Geometry check sheet. Reference: the model listing, model coordinates, mm. A direction names the side the tool comes from. Round coordinates to 2 decimals unless told otherwise and drop trailing zeros. Order: outer loops, then holes, each group sorted by start corner. A loop starts at its lowest first (then second) coordinate and runs counter-clockwise, first axis right, second up. Notation, with made-up numbers: (89.25, -24.75) - (139.25, -24.75) arc R21 cw to (139.25, -12.75) - close; hole circle Ø11 at (34.5, 39.25). An arc over 180 degrees is marked (long way). Use a Markdown table: item, result. Add a question column.
(1) Section check A-A on y = 25. Record the boundary of the cut face in (x, z).
(2) Gauge pin test, flat end, axial feed: P1, Ø2, axis at x = 4, z = 1, coming from the -Y side. Record the tip position at first contact, or that the pin passes through.
(3) Access from +Z, -Z, +X, -X, +Y, -Y to the whole of each face (thin tool, end or side, straight path). Record for faces 5 (the face through (3.035, 48.536, 0.325)), 6 (the face through (1, 52, 0)).
(4) Section check B-B on x = 2.95. Record the boundary of the cut face in (y, z), then the cut area to 3 significant figures.
(5) Mould release check, pull along Y, two halves, no side actions. Record for faces 1 (the face through (4.593, 48.226, -0.923)), 2 (the face through (0.986, 24.571, -1.437)), 3 (the face through (1, -50, 0)), 4 (the face through (1, 38, 2)): released by +Y, released by -Y, zero draft, split by the parting line, or undercut.
(6) Thickness scan on line 1 along Y through (x, z) = (1.55, 0); line 2 along X through (y, z) = (11.5, 0.6); line 3 along Z through (x, y) = (1.3, 25). Record the ranges inside material, lowest first. Write a range as [from, to].
(7) Section check C-C on y = 0.5. Record the boundary of the cut face in (x, z).
```python
from build123d import *

# Parameters (mm, degrees)
BASE_DEPTH         = 2
ESQUISSE2_R        = 1.5
BOSS_FIX_DEPTH     = 2.1
ESQUISSE3_R        = 2
BOSS_BLOCAGE_DEPTH = 1
VIDE_TIGE_DEPTH    = 2
CONGE_TIGE_R       = 0.2


with BuildPart() as part:
    # Esquisse1 → BASE (new body)
    with BuildSketch(Plane(origin=(0, 0, 0), x_dir=(0, 0, -1), z_dir=(1, 0, 0))):
        with BuildLine():
            Line((2, 50), (2, -50))
            Line((2, -50), (-2, -50))
            Line((-2, -50), (-2, 50))
            ThreePointArc((-2, 50), (0, 52), (2, 50))
        make_face()
    extrude(amount=BASE_DEPTH)

    # Esquisse2 → BOSS FIX (add)
    with BuildSketch(Plane(origin=(2, 0, 0), x_dir=(0, 0, -1), z_dir=(1, 0, 0))):
        with Locations((0, 50)):
            Circle(ESQUISSE2_R)
    extrude(amount=BOSS_FIX_DEPTH)

    # Esquisse3 → BOSS BLOCAGE (add)
    with BuildSketch(Plane(origin=(4.1, 0, 0), x_dir=(0, 0, -1), z_dir=(1, 0, 0))):
        with Locations((0, 50)):
            Circle(ESQUISSE3_R)
    extrude(amount=BOSS_BLOCAGE_DEPTH)

    # Esquisse4 → VIDE TIGE (cut)
    with BuildSketch(Plane.ZY):
        with BuildLine():
            Line((0.225177093, 26.483002116), (2, 26))
            Line((2, 26), (2, 24))
            Line((2, 24), (0.937042571, 23.828696786))
            ThreePointArc((0.937042571, 23.828696786), (-1.448800481, 24.611442197), (0.225177093, 26.483002116))
        make_face()
    extrude(amount=-VIDE_TIGE_DEPTH, mode=Mode.SUBTRACT)

    # CONGE TIGE
    conge_tige_edges = [part.edges().sort_by_distance(p)[0] for p in [
        (1, 24, 2),
        (1, 26, 2),
    ]]
    fillet(conge_tige_edges, radius=CONGE_TIGE_R)


solid = part.part
```
Check sheet entries:
| question | item | result |
|---|---|---|
| 1 | outline | (0, -2) - (2, -2) - (2, -1.5) - (0, -1.5) - close |
| 2 | P1 | stops at y = 48 |
| 3 | face 5 | none |
| 3 | face 6 | +X, -X, +Y |
| 4 | outline | circle Ø3 at (50, 0) |
| 4 | area | 7.07 mm2 |
| 5 | face 1 | split by the parting line |
| 5 | face 2 | undercut |
| 5 | face 3 | released by -Y |
| 5 | face 4 | zero draft |
| 6 | line 1 | y = [-50, 23.5], [26.5, 52] |
| 6 | line 2 | x = [0, 2] |
| 6 | line 3 | z = [-2, -1.5] |
| 7 | outline | (0, -2) - (2, -2) - (2, 2) - (0, 2) - close |
